Model file for the job. Use its own axes, mm. Face numbers are marked on the shaded views. A direction names the side the tool comes from. Coordinates: 2 decimals unless noted, no trailing zeros. Order: outer loops, then holes, each group sorted by start corner. A loop starts at its lowest first (then second) coordinate and runs counter-clockwise, first axis right, second up. Notation, with made-up numbers: M 12,-6 L 35,-6 A17 cw 35,2 Z; hole C -21,53.25 d8. An arc over 180 degrees is marked long. Return JSON: item names as keys, results as strings.
```python
from build123d import *

# Parameters (mm, degrees)
BOSS_EXTRUDE1_DEPTH = 50


with BuildPart() as part:
    # Sketch1 → Boss-Extrude1 (new body)
    with BuildSketch(Plane.XY):
        with BuildLine():
            Line((-6.586608294, 14.460119027), (-9.534784216, 15.886812091))
            Line((-9.534784216, 15.886812091), (-15.291700897, 15.886812091))
            Line((-15.291700897, 15.886812091), (-15.291700897, 19.310099191))
            Line((-15.291700897, 19.310099191), (-9.534784216, 19.310099191))
            Line((-9.534784216, 19.310099191), (-5.244334477, 17.233847622))
            ThreePointArc((-5.244334477, 17.233847622), (-1.849307759, 11.35362893), (-3.606603855, 4.795040003))
            ThreePointArc((-3.606603855, 4.795040003), (1.009509443, -5.914464531), (1.811864615, 5.719890438))
            ThreePointArc((1.811864615, 5.719890438), (2.300023264, 12.537382377), (7.465898335, 17.012896867))
            Line((7.465898335, 17.012896867), (9.956628937, 18.439589931))
            Line((9.956628937, 18.439589931), (15.176123212, 18.439589931))
            Line((15.176123212, 18.439589931), (15.176123212, 15.886812091))
            Line((15.176123212, 15.886812091), (9.956628937, 15.886812091))
            Line((9.956628937, 15.886812091), (7.465898335, 14.460119027))
            ThreePointArc((7.465898335, 14.460119027), (4.624724664, 11.219877568), (4.906908203, 6.919667691))
            ThreePointArc((4.906908203, 6.919667691), (-0.457047842, -8.470575915), (-4.133856573, 7.407481279))
            ThreePointArc((-4.133856573, 7.407481279), (-3.899583331, 11.441781667), (-6.586608294, 14.460119027))
        make_face()
    extrude(amount=-BOSS_EXTRUDE1_DEPTH)


solid = part.part
```
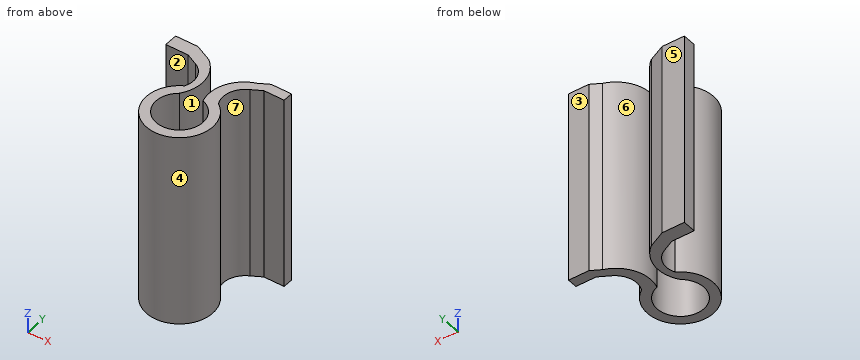
Item 1: Drop flat-ended pins along their axis: pin 1 Ø4 at (y, z) = (10, -17.5) entering from +X; pin 2 Ø3 at (y, z) = (6, -35) entering from -X; pin 3 Ø3 at (x, z) = (-11, -34.5) entering from -Y; pin 4 Ø2 at (x, y) = (3.5, 3) entering from +Z. Give the stop position or say it passes through.
Check result:
{"pin 1": "stops at x = 4.96", "pin 2": "stops at x = -7.19", "pin 3": "stops at y = 15.87", "pin 4": "passes through"}
Item 2: Saw through at C-C (y = 11). Write the cut outline in (x, z).
Check result:
{"outline": "M -3.77,-50 L -1.81,-50 L -1.81,0 L -3.77,0 Z; M 1.7,-50 L 4.56,-50 L 4.56,0 L 1.7,0 Z"}
Item 3: Saw through at D-D (z = -44). Write the cut outline in (x, y), and give its area (3 significant figures).
Check result:
{"outline": "M -15.29,15.89 L -9.53,15.89 L -6.59,14.46 A5.28 cw -4.13,7.41 A8.48 ccw long 4.91,6.92 A5.63 cw 7.47,14.46 L 9.96,15.89 L 15.18,15.89 L 15.18,18.44 L 9.96,18.44 L 7.47,17.01 A8.93 ccw 1.81,5.72 A6 cw long -3.61,4.8 A8.87 ccw -5.24,17.23 L -9.53,19.31 L -15.29,19.31 Z", "area": "201 mm2"}
Item 4: Wall check: line 1 (Y direction, x = 5.5, z = -25); line 2 (X direction, y = 0, z = -23); line 3 (Y direction, x = 0, z = -25). Give the ranges that are in metal, low to high.
Check result:
{"line 1": "y = -6.46 to -2.4, 2.4 to 6.46, 12.85 to 16.08", "line 2": "x = -8.48 to -6, 6 to 8.48", "line 3": "y = -8.48 to -6"}
Item 5: Saw through at B-B (x = 11). Write the cut outline in (y, z), and give its area (3 significant figures).
Check result:
{"outline": "M 15.89,-50 L 18.44,-50 L 18.44,0 L 15.89,0 Z", "area": "128 mm2"}
Item 6: Pull direction X, two halves, no side cores. Call the marked faces 4, 5, 6 and 7: +X half, -X half, draft (parallel to the pull), parting line (faces both ways), or undercut.
Check result:
{"face 4": "parting line", "face 5": "draft", "face 6": "undercut", "face 7": "+X half"}
Item 7: 3-axis set-ups, long thin cutter, end or side, ignore diameter. For the marked faces 1, 2 and 3: which of +Z, -Z, +X, -X, +Y, -Y reach the whole face in a straight line?
Check result:
{"face 1": "+Z, -Z", "face 2": "+Z, -Z, -X, -Y", "face 3": "+Z, -Z, +X, +Y"}
Item 8: Saw through at A-A (y = 0). Write the cut outline in (x, z).
Check result:
{"outline": "M -8.48,-50 L -6,-50 L -6,0 L -8.48,0 Z; M 6,-50 L 8.48,-50 L 8.48,0 L 6,0 Z"}
